The model under review builds one solid part; all positions refer to its coordinate system, in mm. Face numbers are marked on the shaded views. Coordinates: 2 decimals unless noted, no trailing zeros. Order: outer loops, then holes, each group sorted by start corner. A loop starts at its lowest first (then second) coordinate and runs counter-clockwise, first axis right, second up. Notation, with made-up numbers: M 71.25,18 L 79.25,18 A29 ccw 79.25,46 Z; hole C 17.5,85 d6. An arc over 180 degrees is marked long. Write each question's results on one line, items separated by ' | '.
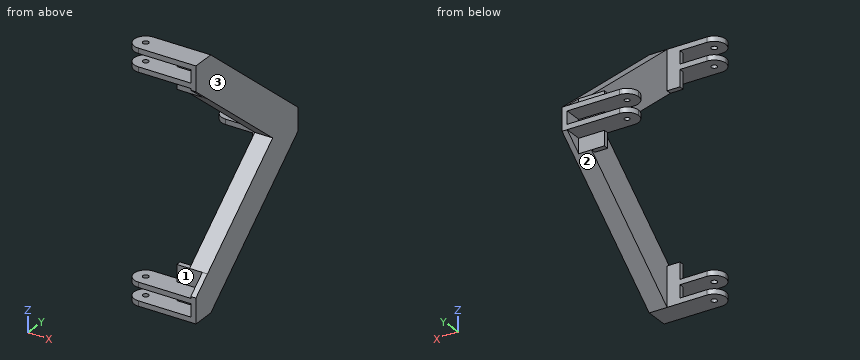
from build123d import *

# Parameters (mm, degrees)
BOSS_EXTRUDE1_DEPTH     = 100
BOSS_EXTRUDE1_2_DEPTH   = 100
BOSS_EXTRUDE1_3_DEPTH   = 100
SKETCH2_W               = 20
SKETCH2_H               = 90
BOSS_EXTRUDE2_DEPTH     = 150
BOSS_EXTRUDE3_DEPTH     = 20
SKETCH4_R               = 11.5
SKETCH4_R_2             = 10
CUT_EXTRUDE2_DEPTH      = 1
CUT_EXTRUDE2_DEPTH_BACK = 966
BOSS_EXTRUDE4_DEPTH     = 50
BOSS_EXTRUDE5_DEPTH     = 10


with BuildPart() as part:
    # Sketch1 → Boss-Extrude1 (new body)
    with BuildSketch(Plane(origin=(0, 0, 0), x_dir=(0, 0, -1), z_dir=(1, 0, 0))):
        Polygon((-462.5, 0), (-412.5, 0), (-412.5, -70), (-392.5, -70), (-392.5, 0), (-327.5, 0), (-327.5, 20), (-482.5, 20), (-482.5, -70), (-462.5, -70), align=None)
    extrude(amount=BOSS_EXTRUDE1_DEPTH)



with BuildPart() as body_2:
    # Sketch1 → Boss-Extrude1 2 (new body)
    with BuildSketch(Plane(origin=(0, 0, 0), x_dir=(0, 0, -1), z_dir=(1, 0, 0))):
        Polygon((25, 477), (-25, 477), (-25, 547), (-45, 547), (-45, 477), (-103.111954459, 477), (-103.111954459, 457), (103.111954459, 457), (103.111954459, 477), (45, 477), (45, 547), (25, 547), align=None)
    extrude(amount=BOSS_EXTRUDE1_2_DEPTH)


with BuildPart() as body_3:
    # Sketch1 → Boss-Extrude1 3 (new body)
    with BuildSketch(Plane(origin=(0, 0, 0), x_dir=(0, 0, -1), z_dir=(1, 0, 0))):
        Polygon((392.5, 0), (327.5, 0), (327.5, 20), (482.5, 20), (482.5, -70), (462.5, -70), (462.5, 0), (412.5, 0), (412.5, -70), (392.5, -70), align=None)
    extrude(amount=BOSS_EXTRUDE1_3_DEPTH)


with BuildPart() as part_1:
    add(part.part)

    add(body_2.part)  # Boss-Extrude2 merges body 2

    add(body_3.part)  # Boss-Extrude2 merges body 3
    # Sketch2 → Boss-Extrude2 (add)
    with BuildSketch(Plane.ZY):
        with Locations((-472.5, -25)):
            Rectangle(SKETCH2_W, SKETCH2_H)
        with Locations((-402.5, -25)):
            Rectangle(SKETCH2_W, SKETCH2_H)
        with Locations((-35, 502)):
            Rectangle(SKETCH2_W, SKETCH2_H)
        with Locations((35, 502)):
            Rectangle(SKETCH2_W, SKETCH2_H)
        with Locations((402.5, -25)):
            Rectangle(SKETCH2_W, SKETCH2_H)
        with Locations((472.5, -25)):
            Rectangle(SKETCH2_W, SKETCH2_H)
    extrude(amount=BOSS_EXTRUDE2_DEPTH)

    # Sketch3 → Boss-Extrude3 (add)
    with BuildSketch(Plane(origin=(100, 0, 0), x_dir=(0, 0, -1), z_dir=(1, 0, 0))):
        Polygon((-482.5, -70), (-482.5, 20), (-45, 547), (45, 547), (482.5, 20), (482.5, -70), (392.5, -70), (385.611954459, -70), (327.5, 0), (0, 394.497142857), (-327.5, 0), (-385.611954459, -70), (-392.5, -70), align=None)
    extrude(amount=BOSS_EXTRUDE3_DEPTH)

    # Sketch4 → Cut-Extrude2 (cut, two sides)
    with BuildSketch(Plane.XY.offset(482.5)) as cut_extrude2_sk:
        with BuildLine():
            ThreePointArc((-150, -25), (-136.819805153, 6.819805153), (-105, 20))
            Line((-105, 20), (-150, 20))
            Line((-150, 20), (-150, -25))
        make_face()
        with Locations((-105, -25)):
            Circle(SKETCH4_R)
        with BuildLine():
            ThreePointArc((-105, -70), (-136.819805153, -56.819805153), (-150, -25))
            Line((-150, -25), (-150, -70))
            Line((-150, -70), (-105, -70))
        make_face()
        with Locations((-105, 502)):
            Circle(SKETCH4_R_2)
        with BuildLine():
            Line((-150, 547), (-150, 502))
            ThreePointArc((-150, 502), (-136.819805153, 533.819805153), (-105, 547))
            Line((-105, 547), (-150, 547))
        make_face()
        with BuildLine():
            Line((-150, 457), (-105, 457))
            ThreePointArc((-105, 457), (-136.819805153, 470.180194847), (-150, 502))
            Line((-150, 502), (-150, 457))
        make_face()
    extrude(amount=CUT_EXTRUDE2_DEPTH, mode=Mode.SUBTRACT)
    extrude(cut_extrude2_sk.sketch, amount=-CUT_EXTRUDE2_DEPTH_BACK, mode=Mode.SUBTRACT)

    # Sketch5 → Boss-Extrude4 (add)
    with BuildSketch(Plane.ZY.offset(-100)):
        Polygon((-482.5, 20), (-103.111954459, 477), (-103.111954459, 461.344354608), (-469.503140685, 20), align=None)
        Polygon((-327.5, 0), (0, 394.497142857), (327.5, 0), (327.5, 15.655645392), (0, 410.15278825), (-327.5, 15.655645392), align=None)
        Polygon((482.5, 20), (469.503140685, 20), (103.111954459, 461.344354608), (103.111954459, 477), align=None)
    extrude(amount=BOSS_EXTRUDE4_DEPTH)

    # Sketch8 → Boss-Extrude5 (add)
    with BuildSketch(Plane.ZY.offset(-50)):
        Polygon((-482.5, 20), (-327.5, 20), (-327.5, 0), (0, 394.497142857), (327.5, 0), (327.5, 20), (482.5, 20), (103.111954459, 477), (-103.111954459, 477), align=None)
    extrude(amount=-BOSS_EXTRUDE5_DEPTH)


solid = part_1.part
1) To check wall thickness, follow line 1 along Y through (x, z) = (-105, -35); line 2 along Y through (x, z) = (-105, 399.75); line 3 along X through (y, z) = (370, 34). State the ranges of each line that lie inside material, in increasing order.
Solutions:
line 1: 457 to 492, 512 to 547 | line 2: -70 to -36.5, -13.5 to 20 | line 3: 50 to 60, 100 to 120
2) For pin 1 (22 mm diameter, centred on y = 6.5, z = -435.5, fed in from -X); pin 2 (4 mm diameter, centred on y = 302.5, z = 153.5, fed in from -X); pin 3 (19.5 mm diameter, centred on x = 75, z = -349, fed in from -Y); pin 4 (19.5 mm diameter, centred on y = -51.5, z = -356, fed in from -X), all flat-tipped, find the tip position at first contact; note any pin that passes through.
Solutions:
pin 1: x = 0 | pin 2: x = 50 | pin 3: y = 0 | pin 4: through
3) The part is to be moulded in two halves that separate along Z. For the marked faces 1, 2 and 3, say which applies: pulls with the +Z half, pulls with the -Z half, needs draft (parallel to the pull), parting line crosses it, or undercut.
Solutions:
face 1: undercut | face 2: pulls with the -Z half | face 3: needs draft
4) Take a section at D-D on z = -123.5. State the section outline as (x, y) points, plus the area to 3 significant figures.
Solutions:
outline: M 50,245.73 L 120,245.73 L 120,452.44 L 50,452.44 Z; hole M 60,261.39 L 100,261.39 L 100,436.79 L 60,436.79 Z | area: 7,450 mm2
5) Take a section at C-C on x = -29.5. State the section outline as (y, z) points.
Solutions:
outline: M -70,-482.5 L 20,-482.5 L 20,-462.5 L -70,-462.5 Z; M -70,-412.5 L 20,-412.5 L 20,-392.5 L -70,-392.5 Z; M -70,392.5 L 20,392.5 L 20,412.5 L -70,412.5 Z; M -70,462.5 L 20,462.5 L 20,482.5 L -70,482.5 Z; M 457,-45 L 547,-45 L 547,-25 L 457,-25 Z; M 457,25 L 547,25 L 547,45 L 457,45 Z
6) Take a section at A-A on x = 22. Count the separate pieces of the cut face and the enclosed holes in it, plus the area to 3 significant figures.
Solutions:
separate pieces: 3 | enclosed holes: 0 | area: 18,700 mm2
7) Take a section at B-B on y = 171. State the section outline as (x, z) points, plus the area to 3 significant figures.
Solutions:
outline: M 50,-357.14 L 120,-357.14 L 120,-185.54 L 50,-185.54 Z; M 50,185.54 L 120,185.54 L 120,357.14 L 50,357.14 Z; hole M 60,-344.15 L 100,-344.15 L 100,-198.54 L 60,-198.54 Z; hole M 60,198.54 L 100,198.54 L 100,344.15 L 60,344.15 Z | area: 12,400 mm2
